Design review of the part shown in the three views and the two pictorial views. Dimensions are in mm from the part's minimum x, y and z. Give positions to 0.01 mm unless a question says otherwise; leave off trailing zeros. Write each loop counter-clockwise with the first axis right and the second up, starting at its lowest first coordinate (ties: lowest second). Pieces come first, ordered by that corner, then holes. Notation, with made-up numbers: M -6.75,-9.75 L 14.25,-9.75 A16 ccw 14.25,-4.75 Z; hole C 28,84 d5. An arc over 180 degrees is marked long. Use one line per item in the form item = value. Start each with the question number.
Q1. Consider section D-D on x = 69. Write out the cut boundary in (y, z), and give its area (3 significant figures).
Q2. Consider section A-A on z = 0.5. Give the number of separate pieces and of enclosed holes in the cut face, and give its area (3 significant figures).
Q3. For probe 1 along Y at (x, z) = (37.5, 1.3); probe 2 along X at (y, z) = (6.25, 0.5); probe 3 along Y at (x, z) = (71, 1.3), list the stretches that pass through material, from the lowest coordinate up. Write a range as [from, to].
Q4. Consider section B-B on x = 37.5. Write out the cut boundary in (y, z), and give its area (3 significant figures).
Q5. Consider section C-C on y = 9. Write out the cut boundary in (x, z), and give its area (3 significant figures).
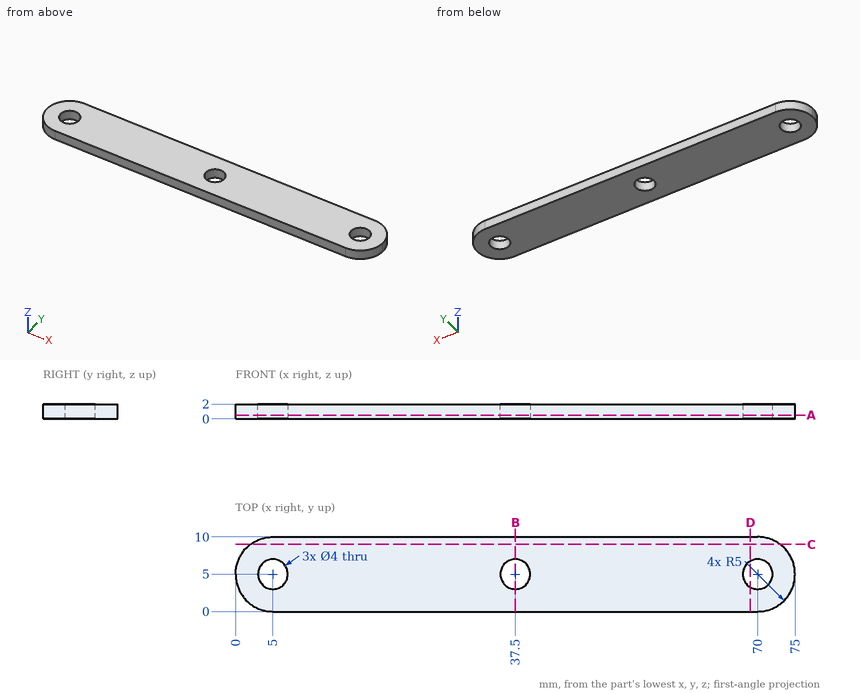
Working result:
q1.outline = M 0,0 L 3.27,0 L 3.27,2 L 0,2 Z; M 6.73,0 L 10,0 L 10,2 L 6.73,2 Z
q1.area = 13.1 mm²
q2.separate_pieces = 1
q2.enclosed_holes = 3
q2.area = 691 mm²
q3.probe_1 = [0, 3], [7, 10]
q3.probe_2 = [0.16, 3.44], [6.56, 35.94], [39.06, 68.44], [71.56, 74.84]
q3.probe_3 = [0.1, 3.27], [6.73, 9.9]
q4.outline = M 0,0 L 3,0 L 3,2 L 0,2 Z; M 7,0 L 10,0 L 10,2 L 7,2 Z
q4.area = 12.0 mm²
q5.outline = M 2,0 L 73,0 L 73,2 L 2,2 Z
q5.area = 142 mm²
